Design review of the part shown in the three views and the two pictorial views. Dimensions are in mm from the part's minimum x, y and z. A direction names the side the tool comes from. Round coordinates to 2 decimals unless told otherwise and drop trailing zeros. Order: outer loops, then holes, each group sorted by start corner. A loop starts at its lowest first (then second) coordinate and runs counter-clockwise, first axis right, second up. Notation, with made-up numbers: (-16.75, 39.25) - (35.25, 39.25) arc R11 cw to (35.25, 49.25) - close; hole circle Ø5 at (-33, -15). An arc over 180 degrees is marked (long way). One line per question, with ' | ' between items. Start each with the question number.
Item 1: Insertion check: pin 1 Ø5 at (x, z) = (2.5, 5.5) entering from -Y; pin 2 Ø5 at (x, z) = (4.5, 11) entering from -Y; pin 3 Ø4 at (x, y) = (4.5, 1) entering from +Z. Each pin has a flat end and moves straight along its axis. Give the tip position at first contact, or say it passes through.
Item 2: Add section B-B on y = 4.15. State the section outline as (x, z) points, and give its area (3 significant figures).
Item 3: Tool access review of the marked faces 5 and 6: name each direction out of +Z, -Z, +X, -X, +Y, -Y from which nothing blocks a thin tool from reaching the whole face with its end or side.
Item 4: Draft analysis for pull direction X (two halves, no side actions). For the marked faces 1, 2, 3 and 4, state which applies: +X half, -X half, draft (parallel to the pull), parting line (faces both ways), or undercut.
Item 5: Add section D-D on z = 8.25. State the section outline as (x, y) points.
Item 6: Add section C-C on x = 4.5. State the section outline as (y, z) points.
Item 7: For L1, parallel to X at y = 1.25, z = 16; L2, parallel to Y at x = 6.8, z = 0.4; L3, parallel to Y at x = 1, z = 5.5, list the stretches that pass through material, from the lowest coordinate up. Write a range as [from, to].
Item 8: Add section A-A on x = 6.8. State the section outline as (y, z) points.
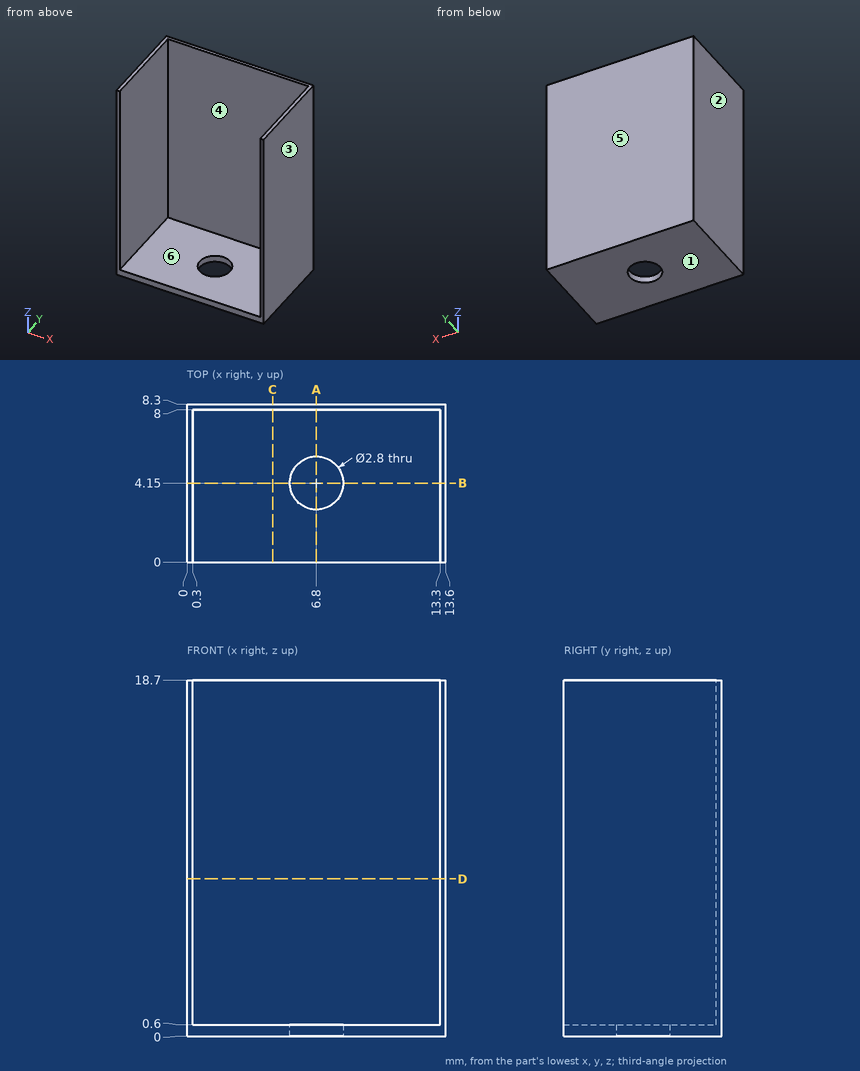
Determined:
1) pin 1: y = 0 | pin 2: y = 8 | pin 3: z = 0.6
2) outline: (0, 0) - (5.4, 0) - (5.4, 0.6) - (0.3, 0.6) - (0.3, 18.7) - (0, 18.7) - close; (8.2, 0) - (13.6, 0) - (13.6, 18.7) - (13.3, 18.7) - (13.3, 0.6) - (8.2, 0.6) - close | area: 17.3 mm2
3) face 5: +Z, -Z, +X, -X, +Y | face 6: +Z, -Y
4) face 1: draft | face 2: -X half | face 3: +X half | face 4: undercut
5) outline: (0, 0) - (0.3, 0) - (0.3, 8) - (13.3, 8) - (13.3, 0) - (13.6, 0) - (13.6, 8.3) - (0, 8.3) - close
6) outline: (0, 0) - (8.3, 0) - (8.3, 18.7) - (8, 18.7) - (8, 0.6) - (0, 0.6) - close
7) L1: [0, 0.3], [13.3, 13.6] | L2: [0, 2.75], [5.55, 8.3] | L3: [8, 8.3]
8) outline: (0, 0) - (2.75, 0) - (2.75, 0.6) - (0, 0.6) - close; (5.55, 0) - (8.3, 0) - (8.3, 18.7) - (8, 18.7) - (8, 0.6) - (5.55, 0.6) - close
